Could you check a few things on this drawing? It's one solid part, dimensions in mm from its lowest x, y, z. A direction names the side the tool comes from. Give positions to 0.01 mm unless a question says otherwise; leave off trailing zeros. Write each loop counter-clockwise with the first axis right and the second up, starting at its lowest first coordinate (ties: lowest second). Pieces come first, ordered by that corner, then holes. Notation, with made-up numbers: M -8.5,3 L 21.5,3 A16 ccw 21.5,13 Z; hole C 86.5,42.5 d3. An arc over 180 degrees is marked long. Write each question's results on one line, items separated by ' | '.
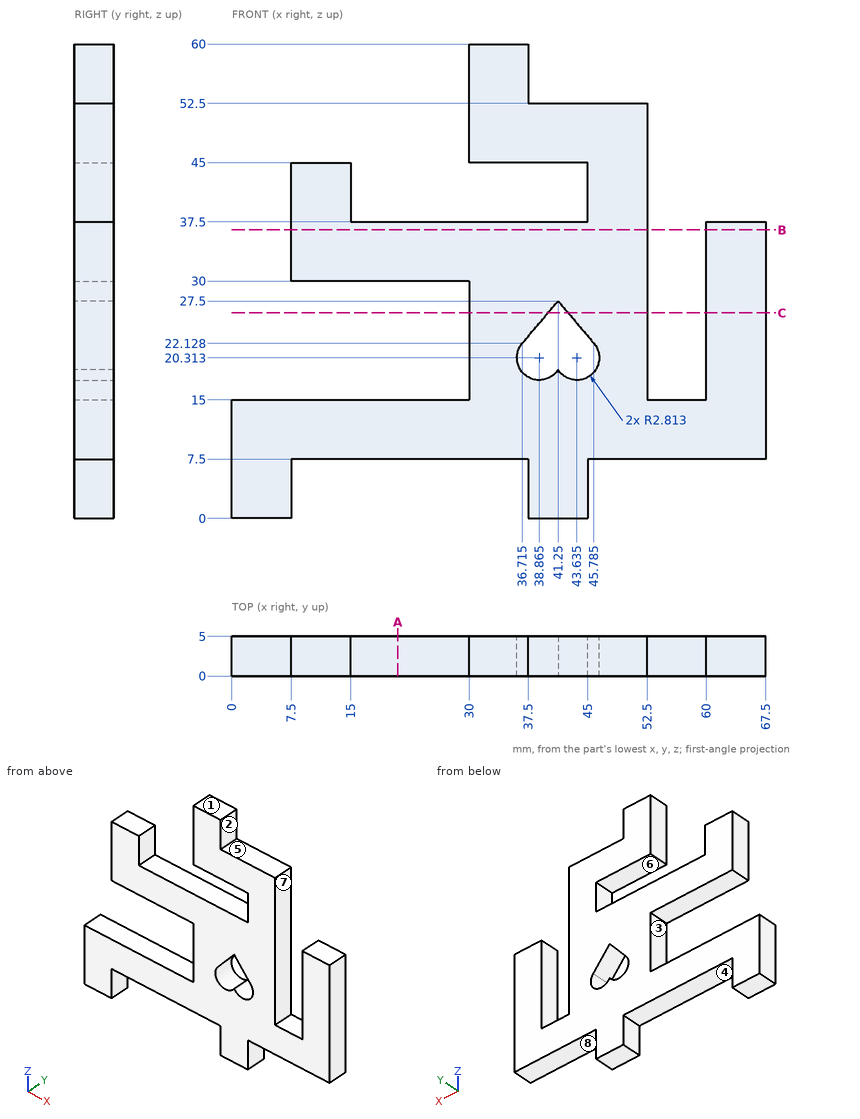
Item 1: I want a section at A-A, the plane x = 21. Please give me the cut outline in (y, z), and give its area (3 significant figures).
Geometry says:
outline: M 0,7.5 L 5,7.5 L 5,15 L 0,15 Z; M 0,30 L 5,30 L 5,37.5 L 0,37.5 Z | area: 75.0 mm2
Item 2: I want a section at B-B, the plane z = 36.5. Please give me the cut outline in (x, y).
Geometry says:
outline: M 7.5,0 L 52.5,0 L 52.5,5 L 7.5,5 Z; M 60,0 L 67.5,0 L 67.5,5 L 60,5 Z
Item 3: I want a section at C-C, the plane z = 26. Please give me the cut outline in (x, y), and give its area (3 significant figures).
Geometry says:
outline: M 30,0 L 39.98,0 L 39.98,5 L 30,5 Z; M 42.52,0 L 52.5,0 L 52.5,5 L 42.52,5 Z; M 60,0 L 67.5,0 L 67.5,5 L 60,5 Z | area: 137 mm2
Item 4: For the marked faces 4, 5, 6, 7 and 8, which set-ups out of +Z, -Z, +X, -X, +Y, -Y let a thin tool reach every point of the face, with its end or its side?
Geometry says:
face 4: -Z, +Y, -Y | face 5: +Z, +X, +Y, -Y | face 6: +Y, -Y | face 7: +Z, +Y, -Y | face 8: -Z, +X, +Y, -Y
Item 5: If I drill on line 1 (X direction, y = 1.35, z = 41.5); line 2 (Z direction, x = 41.5, y = 4.25) (1 decimal); line 3 (X direction, y = 2.1, z = 24) (1 decimal), over which ranges is the centre line in solid material (lowest first)? Write a range as from..to.
Geometry says:
line 1: x = 7.5..15, 45..52.5 | line 2: z = 0..18.5, 27.2..37.5, 45..52.5 | line 3: x = 30..38.3, 44.2..52.5, 60..67.5
Item 6: Thinking about a two-plate mould opening in Z: for the marked faces 1, 2 and 3, which applies, +Z half, -Z half, draft (parallel to the pull), parting line (faces both ways), or undercut?
Geometry says:
face 1: +Z half | face 2: draft | face 3: undercut
Item 7: I'm going to push flat-ended pins straight in: pin 1 (1 mm diameter, centred on x = 33.5, y = 3, fed in from -Z); pin 2 (3 mm diameter, centred on y = 2.5, z = 25, fed in from -X); pin 3 (1 mm diameter, centred on x = 56, z = 6, fed in from -Y); pin 4 (2.5 mm diameter, centred on x = 36.5, y = 2, fed in from -Z). Where does each tip first touch, or does it pass through?
Geometry says:
pin 1: stops at z = 7.5 | pin 2: stops at x = 30 | pin 3: passes through | pin 4: stops at z = 0
